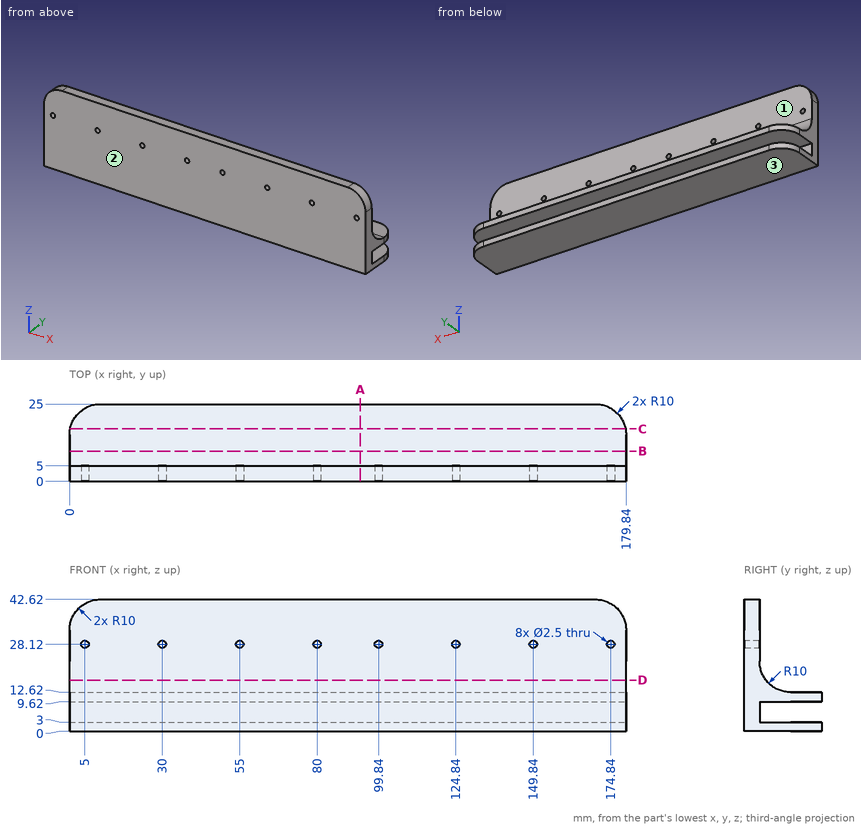
Here's the drawing with two shaded views (mm, measured from the low corner). I have some questions. Coordinates: 2 decimals unless noted, no trailing zeros. Loops run counter-clockwise (first coordinate to the right, second up) from the corner with the lowest first, then second, coordinate; pieces in that order, holes last. Notation, with made-up numbers: (7.25, -29) - (39.25, -29) arc R26 cw to (39.25, -11) - close; hole circle Ø5 at (87, 52). An arc over 180 degrees is marked (long way). Answer as CSV lines item,"result". Start each with the question number.
1) Suppose I cut it at B-B (y = 9.75). Please give me the cut outline in (x, z), plus the area to 3 significant figures.
2) Suppose I cut it at D-D (z = 16.5). Please give me the cut outline in (x, y), plus the area to 3 significant figures.
3) Suppose I cut it at A-A (x = 94). Please give me the cut outline in (y, z).
4) Suppose I cut it at C-C (y = 17). Please give me the cut outline in (x, z).
5) For pin 1 (10 mm diameter, centred on x = 66, z = 8, fed in from +Y); pin 2 (2 mm diameter, centred on x = 55, z = 28.12, fed in from -Y); pin 3 (3 mm diameter, centred on x = 83.5, y = 19.5, fed in from +Z); pin 4 (3.5 mm diameter, centred on x = 80.5, z = 6.5, fed in from +Y), each with a flat end and sliding along its axis, tell me the tip position at first contact or that it passes through.
6) I need wall thicknesses on line 1 (Z direction, x = 111, y = 21.5); line 2 (Z direction, x = 80, y = 3.3); line 3 (Y direction, x = 163, z = 27). Which ranges of each line are inside material? Lowest first, please. Write a range as from..to.
7) Thinking about a two-plate mould opening in Y: for the marked faces 1, 2 and 3, which applies, pulls with the +Y half, pulls with the -Y half, needs draft (parallel to the pull), parting line crosses it, or undercut?
Check result:
1,outline,"(0, 0) - (179.84, 0) - (179.84, 3) - (0, 3) - close; (0, 9.62) - (179.84, 9.62) - (179.84, 14.11) - (0, 14.11) - close"
1,area,"1,350 mm²"
2,outline,"(0, 0) - (179.84, 0) - (179.84, 7.09) - (0, 7.09) - close"
2,area,"1,280 mm²"
3,outline,"(0, 0) - (25, 0) - (25, 3) - (5, 3) - (5, 9.62) - (25, 9.62) - (25, 12.62) - (15, 12.62) arc R10 cw to (5, 22.62) - (5, 42.62) - (0, 42.62) - close"
4,outline,"(0.2, 0) - (179.64, 0) - (179.64, 3) - (0.2, 3) - close; (0.2, 9.62) - (179.64, 9.62) - (179.64, 12.62) - (0.2, 12.62) - close"
5,pin 1,"stops at y = 25"
5,pin 2,"passes through"
5,pin 3,"stops at z = 12.62"
5,pin 4,"stops at y = 5"
6,line 1,"z = 0..3, 9.62..12.62"
6,line 2,"z = 0..26.87, 29.37..42.62"
6,line 3,"y = 0..5"
7,face 1,"pulls with the +Y half"
7,face 2,"pulls with the -Y half"
7,face 3,"needs draft"
